The model under review builds one solid part; all positions refer to its coordinate system, in mm. Round coordinates to 2 decimals unless told otherwise and drop trailing zeros. Write each loop counter-clockwise with the first axis right and the second up, starting at its lowest first coordinate (ties: lowest second). Pieces come first, ordered by that corner, then holes. Notation, with made-up numbers: (53.25, 33.25) -> (65.25, 33.25) arc R4 ccw to (65.25, 37.25) -> close; hole circle Ø2 at (7.5, 53). An arc over 180 degrees is marked (long way). Use CSV: the item, a comma, the result in double quotes. Start each with the question number.
1) Take a section at B-B, the plane z = 185. Give the boundary of the cut face in (x, y).
2) Wall thickness on probe 1 along Y at (x, z) = (0.75, 312.5); probe 2 along Y at (x, z) = (-0.5, 204.5); probe 3 along X at (y, z) = (-0.75, 101): over which ranges is each line inside the solid? List them lowest first. Write a range as [from, to].
3) Take a section at A-A, the plane z = 320. Give the boundary of the cut face in (x, y).
4) For pin 1 Ø1 at (x, z) = (1, 234.5) entering from +Y; pin 2 Ø1.5 at (x, z) = (2.5, 142.5) entering from +Y; pin 3 Ø3 at (y, z) = (-2.5, 189.5) entering from +X, all flat-tipped, find the tip position at first contact; note any pin that passes through.
from build123d import *

# Parameters (mm, degrees)
CROQUIS1_R              = 3.99
SALIENTE_EXTRUIR1_DEPTH = 355
CROQUIS2_W              = 1
CROQUIS2_H              = 0.8
CROQUIS5_R              = 3.99
CROQUIS5_R_2            = 3.96875
CORTAR_EXTRUIR1_DEPTH   = 84
CROQUIS6_R              = 3.99
CROQUIS6_R_2            = 3.97
CORTAR_EXTRUIR2_DEPTH   = 84
CHAFL_N1_SIZE           = 0.5


with BuildPart() as part:
    # Croquis1 → Saliente-Extruir1 (new body)
    with BuildSketch(Plane.XY):
        Circle(CROQUIS1_R)
    extrude(amount=SALIENTE_EXTRUIR1_DEPTH)

    # Croquis2 → Cortar-Revolución1 (revolve, cut)
    with BuildSketch(Plane(origin=(0, 0, 0), x_dir=(0, 0, -1), z_dir=(1, 0, 0))):
        with Locations((-6.5, 3.59)):
            Rectangle(CROQUIS2_W, CROQUIS2_H)
        with Locations((-74.5, 3.59)):
            Rectangle(CROQUIS2_W, CROQUIS2_H)
        with Locations((-83.5, 3.59)):
            Rectangle(CROQUIS2_W, CROQUIS2_H)
    cortar_revoluci_n1 = revolve(axis=Axis((0, 0, 355), (0, 0, -1)), mode=Mode.SUBTRACT)

    # Simetría1: Cortar-Revolución1 across plane
    add(cortar_revoluci_n1.mirror(Plane.XY.offset(177.5)), mode=Mode.SUBTRACT)

    # Croquis5 → Cortar-Extruir1 (cut)
    with BuildSketch(Plane.XY.offset(355)):
        Circle(CROQUIS5_R)
        Circle(CROQUIS5_R_2, mode=Mode.SUBTRACT)
    extrude(amount=-CORTAR_EXTRUIR1_DEPTH, mode=Mode.SUBTRACT)

    # Croquis6 → Cortar-Extruir2 (cut)
    with BuildSketch(Plane(origin=(0, 0, 0), x_dir=(-1, 0, 0), z_dir=(0, 0, -1))):
        Circle(CROQUIS6_R)
        Circle(CROQUIS6_R_2, mode=Mode.SUBTRACT)
    extrude(amount=-CORTAR_EXTRUIR2_DEPTH, mode=Mode.SUBTRACT)

    # Chaflán1
    chafl_n1_edges = [part.edges().sort_by_distance(p)[0] for p in [
        (-3.96875, 0, 355),
        (3.97, 0, 0),
    ]]
    chamfer(chafl_n1_edges, length=CHAFL_N1_SIZE)


solid = part.part
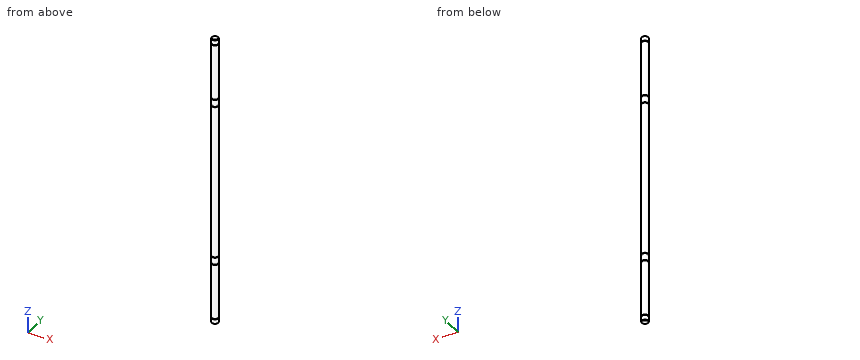
Values found:
1,outline,"circle Ø7.98 at (0, 0)"
2,probe 1,"[-3.9, 3.9]"
2,probe 2,"[-3.96, 3.96]"
2,probe 3,"[-3.92, 3.92]"
3,outline,"circle Ø7.94 at (0, 0)"
4,pin 1,"y = 3.96"
4,pin 2,"y = 3.59"
4,pin 3,"x = 3.86"
